Geometry check sheet. Reference: the model listing, model coordinates, mm. Face numbers are marked on the shaded views. A direction names the side the tool comes from. Give positions to 0.01 mm unless a question says otherwise; leave off trailing zeros. Write each loop counter-clockwise with the first axis right and the second up, starting at its lowest first coordinate (ties: lowest second). Pieces come first, ordered by that corner, then holes.
(1) Thickness scan on line 1 along Y through (x, z) = (0, 12); line 2 along Y through (x, z) = (-7.5, 4.5); line 3 along Z through (x, y) = (18.5, 1.75). Record the ranges inside material, lowest first.
(2) Cross-section at A-A (z = 12). Record the boundary of the cut face in (x, y), and give its area (3 significant figures).
(3) Tool access check on the marked faces 1, 2 and 3. Record the directions out of +Z, -Z, +X, -X, +Y, -Y that give a thin tool (end or side, any length) a straight path to the whole face; none if there is none.
(4) Cross-section at B-B (y = 9.4). Record the boundary of the cut face in (x, z).
(5) Cross-section at C-C (y = 1.5). Record the boundary of the cut face in (x, z), and give its area (3 significant figures).
(6) Cross-section at D-D (x = -5). Record the boundary of the cut face in (y, z), and give its area (3 significant figures).
(7) Depth check by flat-ended pin: P1, Ø9.5, axis at x = -4.5, z = -0.5, coming from the +Y side; P2, Ø0.7, axis at y = 1.5, z = 4.5, coming from the -X side; P3, Ø1.9, axis at y = 1.5, z = -2.5, coming from the +X side; P4, Ø4, axis at x = -8.5, z = -9, coming from the -Y side. Enter the tip coordinate at first touch or a pass-through.
```python
from build123d import *

# Parameters (mm, degrees)
SKETCH1_W           = 18
SKETCH1_H           = 32
SKETCH1_W_2         = 12
SKETCH1_H_2         = 6
BOSS_EXTRUDE1_DEPTH = 2.4
SKETCH4_W           = 1.6
SKETCH4_H           = 8
BOSS_EXTRUDE3_DEPTH = 14
CUT_EXTRUDE2_REACH  = 23.8
SKETCH5_R           = 2.25


with BuildPart() as part:
    # Sketch1 → Boss-Extrude1 (new body)
    with BuildSketch(Plane(origin=(0, 0, 0), x_dir=(1, 0, 0), z_dir=(0, 1, 0))):
        Rectangle(SKETCH1_W, SKETCH1_H)
        with Locations((-15, 13)):
            Rectangle(SKETCH1_W_2, SKETCH1_H_2)
        with Locations((15, 13)):
            Rectangle(SKETCH1_W_2, SKETCH1_H_2)
    extrude(amount=BOSS_EXTRUDE1_DEPTH)

    # Sketch4 → Boss-Extrude3 (add)
    with BuildSketch(Plane(origin=(0, 2.4, 0), x_dir=(1, 0, 0), z_dir=(0, 1, 0))):
        with Locations((0, -12)):
            Rectangle(SKETCH4_W, SKETCH4_H)
    extrude(amount=BOSS_EXTRUDE3_DEPTH)

    # Sketch5 → Cut-Extrude2 (cut, up to next)
    with BuildSketch(Plane.ZY.offset(0.8), mode=Mode.PRIVATE) as cut_extrude2_sk1:
        with Locations((12, 9.4)):
            Circle(SKETCH5_R)
    cut_extrude2_tool1 = extrude(cut_extrude2_sk1.sketch, amount=-CUT_EXTRUDE2_REACH, mode=Mode.PRIVATE) & part.part
    add(cut_extrude2_tool1.solids().sort_by_distance((-0.8, 9.4, 12))[0], mode=Mode.SUBTRACT)


solid = part.part
```
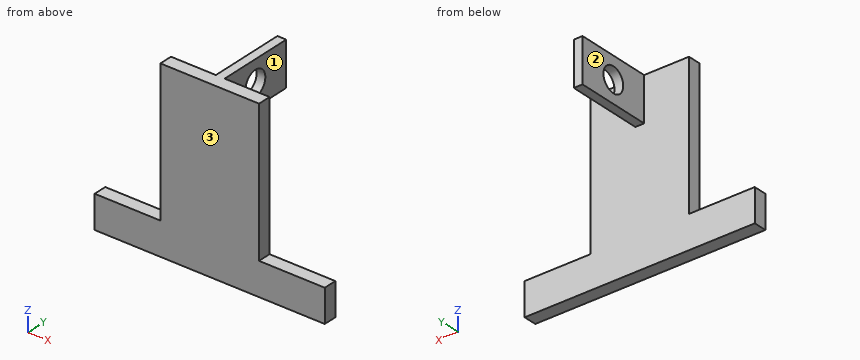
Reply:
1. line 1: y = 0 to 7.15, 11.65 to 16.4
1. line 2: y = 0 to 2.4
1. line 3: z = -16 to -10
2. outline: (-9, 0) - (9, 0) - (9, 2.4) - (0.8, 2.4) - (0.8, 7.15) - (-0.8, 7.15) - (-0.8, 2.4) - (-9, 2.4) - close; (-0.8, 11.65) - (0.8, 11.65) - (0.8, 16.4) - (-0.8, 16.4) - close
2. area: 58.4 mm2
3. face 1: +Z, -Z, +X, +Y
3. face 2: +Z, -Z, -X, +Y
3. face 3: +Z, -Z, +X, -X, -Y
4. outline: (-0.8, 8) - (0.8, 8) - (0.8, 9.75) - (-0.8, 9.75) - close; (-0.8, 14.25) - (0.8, 14.25) - (0.8, 16) - (-0.8, 16) - close
5. outline: (-21, -16) - (21, -16) - (21, -10) - (9, -10) - (9, 16) - (-9, 16) - (-9, -10) - (-21, -10) - close
5. area: 720 mm2
6. outline: (0, -16) - (2.4, -16) - (2.4, 16) - (0, 16) - close
6. area: 76.8 mm2
7. P1: stops at y = 2.4
7. P2: stops at x = -9
7. P3: stops at x = 9
7. P4: stops at y = 0
